The model under review builds one solid part; all positions refer to its coordinate system, in mm. A direction names the side the tool comes from. Coordinates: 2 decimals unless noted, no trailing zeros. Order: outer loops, then holes, each group sorted by start corner. A loop starts at its lowest first (then second) coordinate and runs counter-clockwise, first axis right, second up.
```python
from build123d import *

# Parameters (mm, degrees)
EXTRUDE_1_DEPTH = 4


with BuildPart() as part:
    # 草图1 → 凸台-拉伸1 (new body)
    with BuildSketch(Plane(origin=(0, 0, 0), x_dir=(1, 0, 0), z_dir=(0, 1, 0))):
        with BuildLine():
            Line((-49.404028848, -126.014907086), (-51.26736259, -111.870510049))
            Line((-51.26736259, -111.870510049), (-52.70721139, -111.870510049))
            Line((-52.70721139, -111.870510049), (-59.652364426, -66.218833388))
            Line((-59.652364426, -66.218833388), (-64.988274685, -66.218833388))
            Line((-64.988274685, -66.218833388), (-64.988274685, -68.336258094))
            Line((-64.988274685, -68.336258094), (-68.630245179, -68.336258094))
            Line((-68.630245179, -68.336258094), (-68.630245179, -72.571107506))
            Line((-68.630245179, -72.571107506), (-73.288579532, -72.571107506))
            add(Edge.make_bspline(
                [(-63.143369767, -78.862797811), (-62.992435868, -73.662892561), (-71.907525745, -76.703218171), (-73.288579532, -72.571107506)],
                knots=[0, 0, 0, 0, 1, 1, 1, 1], degree=3))
            Line((-63.143369767, -78.862797811), (-58.583386552, -111.870510049))
            Line((-58.583386552, -111.870510049), (-139.477488779, -111.870510049))
            Line((-139.477488779, -111.870510049), (-134.735106236, -78.862797811))
            add(Edge.make_bspline(
                [(-124.794342828, -72.571107506), (-125.277958037, -74.232765948), (-129.876755781, -75.477760941), (-134.529259996, -75.567175036), (-134.735106236, -78.862797811)],
                knots=[0, 0, 0, 0, 0.392720746, 1, 1, 1, 1], degree=3))
            Line((-124.794342828, -72.571107506), (-128.898327721, -72.571107506))
            Line((-128.898327721, -72.571107506), (-128.898327721, -68.336258094))
            Line((-128.898327721, -68.336258094), (-132.546314293, -68.336258094))
            Line((-132.546314293, -68.336258094), (-132.546314293, -66.218833388))
            Line((-132.546314293, -66.218833388), (-138.291893143, -66.218833388))
            Line((-138.291893143, -66.218833388), (-145.223067629, -111.870510049))
            Line((-145.223067629, -111.870510049), (-146.591062594, -111.870510049))
            Line((-146.591062594, -111.870510049), (-148.232656551, -126.014907086))
            Line((-148.232656551, -126.014907086), (-101.356029105, -126.014907086))
            Line((-101.356029105, -126.014907086), (-101.356029105, -120.624924421))
            Line((-101.356029105, -120.624924421), (-93.356029105, -120.624924421))
            Line((-93.356029105, -120.624924421), (-93.356029105, -126.014907086))
            Line((-93.356029105, -126.014907086), (-49.404028848, -126.014907086))
        make_face()
    extrude(amount=EXTRUDE_1_DEPTH)


solid = part.part
```
(1) We need section D-D, the plane x = -117. Write out the cut boundary in (y, z), and give its area (3 significant figures).
A:
outline: (0, 111.87) - (4, 111.87) - (4, 126.01) - (0, 126.01) - close
area: 56.6 mm2
(2) Draft analysis for pull direction X (two halves, no side actions). For faces 5 (the face through (-131, 2, 68.336)), 6 (the face through (-103, 0, 114)), 7 (the face through (-56.13, 1.97, 89.36)), state which applies: released by +X, released by -X, zero draft, split by the parting line, or undercut.
A:
face 5: undercut
face 6: zero draft
face 7: released by +X
(3) For pin 1 Ø1.2 at (x, y) = (-126, 1.5) entering from -Z; pin 2 Ø2 at (y, z) = (1.5, 122) entering from -X; pin 3 Ø2 at (x, y) = (-96, 1.5) entering from +Z, all flat-tipped, find the tip position at first contact; note any pin that passes through.
A:
pin 1: stops at z = 72.57
pin 2: stops at x = -147.88
pin 3: stops at z = 120.62
(4) Machinability: for faces 1 (the face through (-132.546, 2, 67)), 2 (the face through (-141.71, 1.97, 88.73)), 3 (the face through (-98, 2, 111.871)), 4 (the face through (-101.356, 2, 123)), which of the approach directions +Z, -Z, +X, -X, +Y, -Y give a long, thin tool a straight path to every point of the face, cutting with its end or side? Answer none if there is none.
A:
face 1: -Z, +Y, -Y
face 2: -Z, -X, +Y, -Y
face 3: +Y, -Y
face 4: +Z, +Y, -Y
(5) We need section C-C, the plane z = 103.5. Write out the cut boundary in (x, y), and give its area (3 significant figures).
A:
outline: (-143.95, 0) - (-138.27, 0) - (-138.27, 4) - (-143.95, 4) - close; (-59.74, 0) - (-53.98, 0) - (-53.98, 4) - (-59.74, 4) - close
area: 45.7 mm2
(6) Wall thickness on probe 1 along Z at (x, y) = (-102, 2.6); probe 2 along Z at (x, y) = (-63.5, 1.1); probe 3 along X at (y, z) = (1.35, 89): over which ranges is each line inside the solid? List them lowest first.
A:
probe 1: z = 111.87 to 126.01
probe 2: z = 66.22 to 77.23, 111.87 to 126.01
probe 3: x = -141.75 to -136.19, -61.74 to -56.19
(7) We need section B-B, the plane x = -94.5. Write out the cut boundary in (y, z), and give its area (3 significant figures).
A:
outline: (0, 111.87) - (4, 111.87) - (4, 120.62) - (0, 120.62) - close
area: 35.0 mm2
(8) We need section A-A, the plane z = 84.5. Write out the cut boundary in (x, y), and give its area (3 significant figures).
A:
outline: (-141.07, 0) - (-135.55, 0) - (-135.55, 4) - (-141.07, 4) - close; (-62.36, 0) - (-56.87, 0) - (-56.87, 4) - (-62.36, 4) - close
area: 44.1 mm2
